Read the model definition and answer for the solid it produces. Units are mm, in the model's axes. A direction names the side the tool comes from. Coordinates: 2 decimals unless noted, no trailing zeros. Loops run counter-clockwise (first coordinate to the right, second up) from the corner with the lowest first, then second, coordinate; pieces in that order, holes last.
from build123d import *

# Parameters (mm, degrees)
BOSS_EXTRUDE1_DEPTH = 3
SKETCH2_R           = 11.5
BOSS_EXTRUDE2_DEPTH = 10
SKETCH3_R           = 10.5
CUT_EXTRUDE1_DEPTH  = 10


with BuildPart() as part:
    # Sketch1 → Boss-Extrude1 (new body)
    with BuildSketch(Plane(origin=(0, 0, 0), x_dir=(1, 0, 0), z_dir=(0, 1, 0))):
        Polygon((7.216878365, -12.5), (14.43375673, 0), (7.216878365, 12.5), (-7.216878365, 12.5), (-14.43375673, 0), (-7.216878365, -12.5), align=None)
    extrude(amount=BOSS_EXTRUDE1_DEPTH)

    # Sketch2 → Boss-Extrude2 (add)
    with BuildSketch(Plane(origin=(0, 3, 0), x_dir=(1, 0, 0), z_dir=(0, 1, 0))):
        Circle(SKETCH2_R)
    extrude(amount=BOSS_EXTRUDE2_DEPTH)

    # Sketch3 → Cut-Extrude1 (cut)
    with BuildSketch(Plane(origin=(0, 13, 0), x_dir=(1, 0, 0), z_dir=(0, 1, 0))):
        Circle(SKETCH3_R)
    extrude(amount=-CUT_EXTRUDE1_DEPTH, mode=Mode.SUBTRACT)


solid = part.part
Q1. A cutting plane is placed at C-C (z = 8.75). Give the vertices of the cut face in (x, y), then the cut area to 3 significant figures.
Findings below:
outline: (-9.38, 0) - (9.38, 0) - (9.38, 3) - (7.46, 3) - (7.46, 13) - (5.8, 13) - (5.8, 3) - (-5.8, 3) - (-5.8, 13) - (-7.46, 13) - (-7.46, 3) - (-9.38, 3) - close
area: 89.5 mm2
Q2. A cutting plane is placed at D-D (y = 7). Give the vertices of the cut face in (x, z).
Findings below:
outline: circle Ø23 at (0, 0); hole circle Ø21 at (0, 0)
Q3. A cutting plane is placed at B-B (y = 2.25). Give the vertices of the cut face in (x, z).
Findings below:
outline: (-14.43, 0) - (-7.22, -12.5) - (7.22, -12.5) - (14.43, 0) - (7.22, 12.5) - (-7.22, 12.5) - close
Q4. Straight lines are drawn through the part: probe 1 along Z at (x, y) = (0, 8.75); probe 2 along Y at (x, z) = (1.5, -1). For each, find the intervals that lie inside material, in ascending order.
Findings below:
probe 1: z = -11.5 to -10.5, 10.5 to 11.5
probe 2: y = 0 to 3
Q5. Determine the mould class of faces 3 (the face through (-10.775, 1.479, -6.337)), 4 (the face through (0, 1, 12.5)), 5 (the face through (10, 8.1, -3.2)) for opening direction Z: +Z half, -Z half, draft (parallel to the pull), parting line (faces both ways), or undercut.
Findings below:
face 3: -Z half
face 4: +Z half
face 5: undercut
Q6. Which of the six approach directions +Z, -Z, +X, -X, +Y, -Y give full straight-line access (tool end or side, diameter ignored) to faces 1 (the face through (3.4, 13, 10.2)), 2 (the face through (11, 3, -5))?
Findings below:
face 1: +Z, -Z, +X, -X, +Y
face 2: +Y
Q7. Flat-ended cylindrical pins translate along their axes: pin 1 Ø1 at (x, y) = (4, 6) entering from +Z; pin 2 Ø1.5 at (y, z) = (11, 3.5) entering from -X; pin 3 Ø7.5 at (x, z) = (4.5, 6) entering from +Y; pin 4 Ø6 at (x, y) = (10.5, 6.5) entering from +Z. Find the tip coordinate at first contact, or state that the pin passes through.
Findings below:
pin 1: stops at z = 10.95
pin 2: stops at x = -11.17
pin 3: stops at y = 13
pin 4: stops at z = 8.72
Q8. A cutting plane is placed at A-A (x = 0). Give the vertices of the cut face in (y, z), then the cut area to 3 significant figures.
Findings below:
outline: (0, -12.5) - (3, -12.5) - (3, -11.5) - (13, -11.5) - (13, -10.5) - (3, -10.5) - (3, 10.5) - (13, 10.5) - (13, 11.5) - (3, 11.5) - (3, 12.5) - (0, 12.5) - close
area: 95.0 mm2
